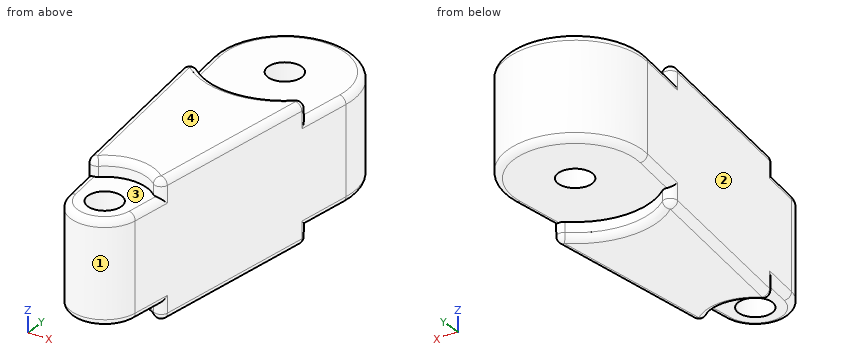
```python
from build123d import *

# Parameters (mm, degrees)
SKETCH1_R            = 6.35
SKETCH1_R_2          = 6.349999999999998
BOSS_EXTRUDE1_DEPTH  = 19.05
BOSS_EXTRUDE2_DEPTH  = 6.35
FILLET1_R            = 2.54
FILLET1_OF_MIRROR4_R = 2.54


with BuildPart() as part:
    # Sketch1 → Boss-Extrude1 (new body)
    with BuildSketch(Plane.XY):
        with BuildLine():
            Line((-25.20078123789022, 98.425), (-12.600390618945115, -1.5875000000000004))
            ThreePointArc((-12.600390618945115, -1.5875000000000004), (7.8e-16, -12.700000000000003), (12.600390618945115, -1.5875000000000004))
            Line((12.600390618945115, -1.5875000000000004), (25.20078123789022, 98.425))
            ThreePointArc((25.20078123789022, 98.425), (-4.67e-15, 126.99999999999999), (-25.20078123789022, 98.425))
        make_face()
        with Locations(Location((0, 0, 0), (0, 0, 180))):
            Circle(SKETCH1_R, mode=Mode.SUBTRACT)
        with Locations(Location((0, 101.6, 0), (0, 0, 180))):
            Circle(SKETCH1_R_2, mode=Mode.SUBTRACT)
    boss_extrude1 = extrude(amount=BOSS_EXTRUDE1_DEPTH)

    # Sketch2 → Boss-Extrude2 (add)
    with BuildSketch(Plane.XY.offset(19.05)):
        with BuildLine():
            Line((-23.56442369272321, 85.43681463851183), (-13.791015618945115, 7.862792964208833))
            ThreePointArc((-13.791015618945114, 7.8627929642088334), (-2.55e-15, 15.875), (13.791015618945112, 7.862792964208835))
            Line((13.791015618945114, 7.862792964208836), (23.56442369272321, 85.43681463851183))
            ThreePointArc((23.564423692723203, 85.43681463851182), (-5.25e-15, 73.02499999999999), (-23.56442369272321, 85.43681463851183))
        make_face()
    boss_extrude2 = extrude(amount=BOSS_EXTRUDE2_DEPTH)

    # Fillet1
    fillet1_edges = [part.edges().sort_by_distance(p)[0] for p in [
        (-2.22e-15, -12.700000000000003, 19.05),
        (13.195703118945115, 3.137646482104417, 19.05),
        (-13.195703118945115, 3.137646482104415, 19.05),
        (24.382602465306718, 91.93090731925592, 19.05),
        (8.9e-16, 15.875000000000002, 25.4),
        (-13.791015618945114, 7.862792964208833, 22.225),
        (13.791015618945114, 7.862792964208834, 22.225),
        (-1.066e-14, 73.02499999999999, 25.4),
        (23.564423692723206, 85.43681463851183, 22.225),
        (-23.564423692723214, 85.43681463851183, 22.225),
        (18.67771965583416, 46.649803801360335, 25.4),
        (-18.677719655834164, 46.649803801360335, 25.4),
        (-3.11e-15, 126.99999999999999, 19.05),
        (-24.382602465306714, 91.93090731925591, 19.05),
    ]]
    fillet(fillet1_edges, radius=FILLET1_R)

    # Mirror4: Boss-Extrude1, Boss-Extrude2 across plane
    add(boss_extrude1.mirror(Plane(origin=(0, 101.6, 0), x_dir=(1, 0, 0), z_dir=(0, 0, -1))))
    add(boss_extrude2.mirror(Plane(origin=(0, 101.6, 0), x_dir=(1, 0, 0), z_dir=(0, 0, -1))))

    # Fillet1 of Mirror4
    fillet1_of_mirror4_edges = [part.edges().sort_by_distance(p)[0] for p in [
        (-2.22e-15, -12.700000000000003, -19.05),
        (13.195703118945115, 3.137646482104417, -19.05),
        (-13.195703118945115, 3.137646482104415, -19.05),
        (24.382602465306718, 91.93090731925592, -19.05),
        (8.9e-16, 15.875000000000002, -25.4),
        (-13.791015618945114, 7.862792964208833, -22.225),
        (13.791015618945114, 7.862792964208834, -22.225),
        (-1.066e-14, 73.02499999999999, -25.4),
        (23.564423692723206, 85.43681463851183, -22.225),
        (-23.564423692723214, 85.43681463851183, -22.225),
        (18.67771965583416, 46.649803801360335, -25.4),
        (-18.677719655834164, 46.649803801360335, -25.4),
        (-3.11e-15, 126.99999999999999, -19.05),
        (-24.382602465306714, 91.93090731925591, -19.05),
    ]]
    fillet(fillet1_of_mirror4_edges, radius=FILLET1_OF_MIRROR4_R)


solid = part.part
```
Can you work these out from the model? Positions are in its coordinate system, mm. Face numbers are marked on the shaded views. Give positions to 0.01 mm unless a question says otherwise; leave off trailing zeros. Order: outer loops, then holes, each group sorted by start corner. A loop starts at its lowest first (then second) coordinate and runs counter-clockwise, first axis right, second up. Notation, with made-up numbers: M 42.25,84.5 L 62.25,84.5 A19 cw 62.25,92.5 Z; hole C -2,-14.75 d6. An arc over 180 degrees is marked long. Write item = value, one per line. Start each with the question number.
Q1. Suppose I cut it at B-B (z = -8). Count the separate pieces of the cut face and the enclosed holes in it, plus the area to 3 significant figures.
Q2. I need wall thicknesses on probe 1 along X at (y, z) = (101.6, -14.75); probe 2 along Z at (x, y) = (5, 121.5); probe 3 along X at (y, z) = (105, 4.5). Which ranges of each line are inside material? Lowest first, please. Write a range as [from, to].
Q3. Suppose I cut it at C-C (y = 101.6). Write out the boundary of the cut face in (x, z), plus the area to 3 significant figures.
Q4. Will these pins go through, and if not, where does the flat tip stop? pin 1 Ø5 at (y, z) = (82, -1.5) entering from +X; pin 2 Ø10 at (x, y) = (0, 101.6) entering from -Z; pin 3 Ø12 at (y, z) = (74, -9.5) entering from -X; pin 4 Ø2 at (x, y) = (5, 95) entering from -Z.
Q5. We'd pull the mould along X, two halves only. Please class the marked faces 1, 2, 3 and 4: pulls with the +X half, pulls with the -X half, needs draft (parallel to the pull), parting line crosses it, or undercut.
Q6. Suppose I cut it at A-A (x = 0). Write out the boundary of the cut face in (y, z) (3 decimals), plus the area to 3 significant figures.
Check result:
q1.separate_pieces = 1
q1.enclosed_holes = 2
q1.area = 4,910 mm2
q2.probe_1 = [-25.4, -6.35], [6.35, 25.4]
q2.probe_2 = [-19.05, 19.05]
q2.probe_3 = [-25.17, -5.36], [5.36, 25.17]
q3.outline = M -25.4,-16.51 A2.54 ccw -22.86,-19.05 L -6.35,-19.05 L -6.35,19.05 L -22.86,19.05 A2.54 ccw -25.4,16.51 Z; M 6.35,-19.05 L 22.86,-19.05 A2.54 ccw 25.4,-16.51 L 25.4,16.51 A2.54 ccw 22.86,19.05 L 6.35,19.05 Z
q3.area = 1,450 mm2
q4.pin_1 = 23.45
q4.pin_2 = through
q4.pin_3 = -22.88
q4.pin_4 = -19.05
q5.face_1 = parting line crosses it
q5.face_2 = pulls with the -X half
q5.face_3 = undercut
q5.face_4 = needs draft
q6.outline = M -12.7,-16.51 A2.54 ccw -10.16,-19.05 L -6.35,-19.05 L -6.35,19.05 L -10.16,19.05 A2.54 ccw -12.7,16.51 Z; M 6.35,-19.05 L 15.875,-19.05 L 15.875,-22.86 A2.54 ccw 18.415,-25.4 L 70.485,-25.4 A2.54 ccw 73.025,-22.86 L 73.025,-19.05 L 95.25,-19.05 L 95.25,19.05 L 73.025,19.05 L 73.025,22.86 A2.54 ccw 70.485,25.4 L 18.415,25.4 A2.54 ccw 15.875,22.86 L 15.875,19.05 L 6.35,19.05 Z; M 107.95,-19.05 L 124.46,-19.05 A2.54 ccw 127,-16.51 L 127,16.51 A2.54 ccw 124.46,19.05 L 107.95,19.05 Z
q6.area = 5,070 mm2
